The model under review builds one solid part; all positions refer to its coordinate system, in mm. A direction names the side the tool comes from. Coordinates: 2 decimals unless noted, no trailing zeros. Write each loop counter-clockwise with the first axis right and the second up, starting at its lowest first coordinate (ties: lowest second). Pieces come first, ordered by that corner, then holes. Notation, with made-up numbers: M 12.25,79 L 71.25,79 A23 cw 71.25,105 Z; hole C 26.25,-7.5 d8. An arc over 180 degrees is marked long. Answer as a JSON object with one key per item and string values.
Autodesk Inventor part; units mm, degrees
ref_plane "YZ Plane" through (0, 0, 0) normal (1, 0, 0) x (0, 1, 0)
ref_plane "XZ Plane" through (0, 0, 0) normal (0, 1, 0) x (-1, 0, 0)
ref_plane "XY Plane" through (0, 0, 0) normal (0, 0, 1) x (1, 0, 0)
sketch "Sketch1" plane through (0, 0, 0) normal (0, 0, 1) x (1, 0, 0)
  line L0 (-34.86, 0) -> (34.86, 0) construction
  line L1 (0, -34.86) -> (0, 34.86) construction
  line L2 (0, 0) -> (16.9726, 16.9726) construction
  line L3 (0, 0) -> (24.0028, 0) construction
  line L4 (0, 24.9) -> (16.8009, 24.9)
  line L5 (16.8009, 24.9) -> (16.8009, 21.2415)
  line L6 (16.8009, 21.2415) -> (19.0212, 19.0212)
  line L7 (24.9, 0) -> (24.9, 16.8009)
  line L8 (24.9, 16.8009) -> (21.2415, 16.8009)
  line L9 (21.2415, 16.8009) -> (19.0212, 19.0212)
  line L10 (0, -24.9) -> (16.8009, -24.9)
  line L11 (16.8009, -24.9) -> (16.8009, -21.2415)
  line L12 (16.8009, -21.2415) -> (19.0212, -19.0212)
  line L13 (24.9, 0) -> (24.9, -16.8009)
  line L14 (24.9, -16.8009) -> (21.2415, -16.8009)
  line L15 (21.2415, -16.8009) -> (19.0212, -19.0212)
  line L16 (0, 0) -> (-16.9726, 16.9726) construction
  line L17 (0, 0) -> (-24.0028, 0) construction
  line L18 (0, 24.9) -> (-16.8009, 24.9)
  line L19 (-16.8009, 24.9) -> (-16.8009, 21.2415)
  line L20 (-16.8009, 21.2415) -> (-19.0212, 19.0212)
  line L21 (-24.9, 0) -> (-24.9, 16.8009)
  line L22 (-24.9, 16.8009) -> (-21.2415, 16.8009)
  line L23 (-21.2415, 16.8009) -> (-19.0212, 19.0212)
  line L24 (0, -24.9) -> (-16.8009, -24.9)
  line L25 (-16.8009, -24.9) -> (-16.8009, -21.2415)
  line L26 (-16.8009, -21.2415) -> (-19.0212, -19.0212)
  line L27 (-21.2415, -16.8009) -> (-19.0212, -19.0212)
  line L28 (-24.9, -16.8009) -> (-21.2415, -16.8009)
  line L29 (-24.9, 0) -> (-24.9, -16.8009)
  circle A0 centre (0, 0) radius 10
  dimension "d17" = 45
  dimension "d18" = 24.9
  dimension "d20" = 3.14
  dimension "d21" = 26.9
  dimension "d22" = 20
extrude "Extrusion1" add sketch "Sketch1" along normal blind 5
sketch "Sketch2" plane through (0, 0, 5) normal (0, 0, 1) x (1, 0, 0)
  circle A0 centre (0, 0) radius 10
  line L0 (16.8009, 24.9) -> (-16.8009, 24.9)
  line L1 (-16.8009, 24.9) -> (-16.8009, 21.2415)
  line L2 (-16.8009, 21.2415) -> (-21.2415, 16.8009)
  line L3 (-21.2415, 16.8009) -> (-24.9, 16.8009)
  line L4 (-24.9, 16.8009) -> (-24.9, -16.8009)
  line L5 (-24.9, -16.8009) -> (-21.2415, -16.8009)
  line L6 (-21.2415, -16.8009) -> (-16.8009, -21.2415)
  line L7 (-16.8009, -21.2415) -> (-16.8009, -24.9)
  line L8 (-16.8009, -24.9) -> (16.8009, -24.9)
  line L9 (16.8009, -24.9) -> (16.8009, -21.2415)
  line L10 (16.8009, -21.2415) -> (21.2415, -16.8009)
  line L11 (21.2415, -16.8009) -> (24.9, -16.8009)
  line L12 (24.9, -16.8009) -> (24.9, 16.8009)
  line L13 (24.9, 16.8009) -> (21.2415, 16.8009)
  line L14 (21.2415, 16.8009) -> (16.8009, 21.2415)
  line L15 (16.8009, 21.2415) -> (16.8009, 24.9)
  line L16 (0, -34.86) -> (0, 34.86) construction
  line L17 (-12, 12) -> (-7, 12)
  line L18 (-7, 12) -> (-7, 10)
  line L19 (-7, 10) -> (-12, 10)
  line L20 (-12, 10) -> (-12, 12)
  dimension "d27" = 2
  dimension "d28" = 5
  dimension "d29" = 12
extrude "Extrusion2" add sketch "Sketch2" along normal blind 21 contours L17 L18 L19 L20
sketch "Sketch4" plane through (-12, 10, 5) normal (-1, 0, 0) x (0, 0, 1)
  line L0 (0, 0) -> (0, 2)
  line L1 (0, 0) -> (21, 0)
  line L2 (21, 2) -> (21, 0)
  line L3 (0, 2) -> (21, 2)
  line L4 (0, 6.8009) -> (0, -26.8009)
  line L5 (0, 2) -> (21, 2)
  line L6 (21, 2) -> (0, 2)
  line L7 (0, 2) -> (0, 6)
  line L8 (0, -26.8009) -> (0, 6.8009)
  line L9 (0, 6) -> (21, 2)
  point P0 (-5, -10)
  dimension "d35" = 4
extrude "Extrusion4" add sketch "Sketch4" against normal up to surface (5 mm away) contours L4 L9 L3
sketch "Sketch5" plane through (-12, 10, 5) normal (0, -1, 0) x (1, 0, 0)
  line L0 (5, 21) -> (5, 0)
  line L1 (0, 0) -> (5, 0)
  line L2 (0, 21) -> (0, 0)
  line L3 (5, 21) -> (0, 21)
  line L4 (12, -10.2) -> (12, 26.2) construction
  line L5 (0, 21) -> (2, 21)
  line L6 (2, 21) -> (2, 0)
  line L7 (2, 0) -> (0, 0)
  line L8 (0, 0) -> (0, 21)
  point P0 (12, -5)
  dimension "d38" = 10
extrude "Extrusion5" add sketch "Sketch5" along normal blind 1 contours L6 L1 L2 L3
mirror "Mirror1" about plane through (0, 0, 0) normal (0, 1, 0) of "Extrusion2", "Extrusion4", "Extrusion5"
mirror "Mirror2" about plane through (0, 0, 0) normal (1, 0, 0) of "Extrusion2", "Extrusion4", "Mirror1", "Extrusion5"
properties part number "20_Cube_Insert_Beamsplitter"
(1) Draft analysis for pull direction X (two halves, no side actions). For faces 6 (the face through (7, -12, 13)), 7 (the face through (-9.54, 14.03, 15.35)), 8 (the face through (12, -12, 13)), state which applies: released by +X, released by -X, zero draft, split by the parting line, or undercut.
Results list:
{"face 6": "undercut", "face 7": "zero draft", "face 8": "released by +X"}
(2) For pin 1 Ø0.8 at (y, z) = (9.5, 13) entering from +X; pin 2 Ø3 at (y, z) = (-23, 2) entering from -X; pin 3 Ø6 at (x, y) = (15, -11.5) entering from -Z; pin 4 Ø8 at (x, z) = (-19, 22) entering from -Y, all flat-tipped, find the tip position at first contact; note any pin that passes through.
Results list:
{"pin 1": "x = 12", "pin 2": "x = -16.8", "pin 3": "z = 0", "pin 4": "through"}
(3) For faces 1 (the face through (11, -9, 16)), 2 (the face through (23, -16.801, 2)), 3 (the face through (12, 12, 13)), 4 (the face through (-16.801, -23, 2)), 5 (the face through (-23, 16.801, 2)), list the 3-axis set-ups (+Z, -Z, +X, -X, +Y, -Y) from which the entire face can be reached by the end or side of a thin tool; tool diameter is ignored.
Results list:
{"face 1": "+Z, +X, -X", "face 2": "+Z, -Z, +X, -Y", "face 3": "+Z, +X, +Y, -Y", "face 4": "+Z, -Z, -X, -Y", "face 5": "+Z, -Z, -X, +Y"}
(4) Add section D-D on y = 13.5. Give the boundary of the cut face in (x, z) (3 decimals).
Results list:
{"outline": "M -24.9,0 L 24.9,0 L 24.9,5 L 12,5 L 12,18.125 L 7,18.125 L 7,5 L -7,5 L -7,18.125 L -12,18.125 L -12,5 L -24.9,5 Z"}
(5) Add section A-A on y = 0. Give the boundary of the cut face in (x, z).
Results list:
{"outline": "M -24.9,0 L -10,0 L -10,5 L -24.9,5 Z; M 10,0 L 24.9,0 L 24.9,5 L 10,5 Z"}
(6) Add section C-C on z = 15. Give the boundary of the cut face in (x, y).
Results list:
{"outline": "M -12,-14.1 L -7,-14.1 L -7,-10 L -10,-10 L -10,-9 L -12,-9 Z; M -12,9 L -10,9 L -10,10 L -7,10 L -7,14.1 L -12,14.1 Z; M 7,-14.1 L 12,-14.1 L 12,-9 L 10,-9 L 10,-10 L 7,-10 Z; M 7,10 L 10,10 L 10,9 L 12,9 L 12,14.1 L 7,14.1 Z"}
(7) Wall thickness on line 1 along Y through (x, z) = (0, 2.65); line 2 along X through (y, z) = (9.5, 20.25); line 3 along Z through (x, y) = (18, 16.5): over which ranges is each line inside the solid? List them lowest first. Write a range as from..to.
Results list:
{"line 1": "-24.9..-10, 10..24.9", "line 2": "-12..-10, 10..12", "line 3": "0..5"}
